Could you check a few things on this model? Use its own coordinates, in mm. A direction names the side the tool comes from. Coordinates: 2 decimals unless noted, no trailing zeros. Order: outer loops, then holes, each group sorted by start corner. A loop starts at its lowest first (then second) coordinate and runs counter-clockwise, first axis right, second up. Notation, with made-up numbers: (-12, 81) - (6, 81) arc R34 cw to (6, 114) - close; hole circle Ø8 at (45.25, 43.25). An arc over 180 degrees is marked (long way). Answer as a JSON object with one key per item and string values. Group by question number.
(1) Imagine slicing it at B-B, the plane x = 0. Write out the boundary of the cut face in (y, z), and give its area (4 significant figures).
(2) Which directions (+Z, -Z, +X, -X, +Y, -Y) give clear straight access to the entire face, cutting with the end or side of a thin tool? Please do faces 5 (the flat face through (0, 1, 3.9)), 6 (the flat face through (8, 1, 5.5)), 7 (the flat face through (-10, 1, -7)).
(3) Imagine slicing it at A-A, the plane z = 0. Write out the boundary of the cut face in (x, y), and give its area (4 significant figures).
(4) Please list where these lines run through material, in increasing order: probe 1 along Z at (x, y) = (-8, -23.5); probe 2 along Z at (x, y) = (9, 34.5); probe 3 along X at (y, z) = (-0.5, 0).
(5) Will these pins go through, and if not, where does the flat tip stop? P1, Ø1.5, axis at x = 0, z = 0, coming from the -Y side; P2, Ø1, axis at x = 2, y = -11, coming from the -Z side.
(6) We'd pull the mould along X, two halves only. Please class faces 1 (the flat face through (2, -57.5, -2)), 2 (the flat face through (-10, 1, 7)), 3 (the flat face through (10, 1, 7)), 4 (the flat face through (5.25, 0.8, 4.19)): pulls with the +X half, pulls with the -X half, needs draft (parallel to the pull), parting line crosses it, or undercut.
from build123d import *

# Parameters (mm, degrees)
SKETCH1_R           = 2.55
BOSS_EXTRUDE1_DEPTH = 57.5


with BuildPart() as part:
    # Sketch1 → Boss-Extrude1 (new, symmetric)
    with BuildSketch(Plane(origin=(0, 0, 0), x_dir=(1, 0, 0), z_dir=(0, 1, 0))):
        Polygon((-6.560660172, 5.5), (-3.9, 2.839339828), (-3.9, -2.839339828), (-6.560660172, -5.5), (-8.5, -5.5), (-8.5, -3.1), (-9.639683838, -3.1), (-9.639683838, -3.65), (-10, -3.65), (-10, -10), (-3.65, -10), (-3.65, -9.639683838), (-3.1, -9.639683838), (-3.1, -8.5), (-5.5, -8.5), (-5.5, -6.560660172), (-2.839339828, -3.9), (2.839339828, -3.9), (5.5, -6.560660172), (5.5, -8.5), (3.1, -8.5), (3.1, -9.639683838), (3.65, -9.639683838), (3.65, -10), (10, -10), (10, -3.65), (9.639683838, -3.65), (9.639683838, -3.1), (8.5, -3.1), (8.5, -5.5), (6.560660172, -5.5), (3.9, -2.839339828), (3.9, 2.839339828), (6.560660172, 5.5), (8.5, 5.5), (8.5, 3.1), (9.639683838, 3.1), (9.639683838, 3.65), (10, 3.65), (10, 10), (3.65, 10), (3.65, 9.639683838), (3.1, 9.639683838), (3.1, 8.5), (5.5, 8.5), (5.5, 6.560660172), (2.839339828, 3.9), (-2.839339828, 3.9), (-5.5, 6.560660172), (-5.5, 8.5), (-3.1, 8.5), (-3.1, 9.639683838), (-3.65, 9.639683838), (-3.65, 10), (-10, 10), (-10, 3.65), (-9.639683838, 3.65), (-9.639683838, 3.1), (-8.5, 3.1), (-8.5, 5.5), align=None)
        with Locations(Location((0, 0, 0), (0, 0, 270))):
            Circle(SKETCH1_R, mode=Mode.SUBTRACT)
    extrude(amount=BOSS_EXTRUDE1_DEPTH, both=True)


solid = part.part
Result set:
{
 "1": {"outline": "(-57.5, -3.9) - (57.5, -3.9) - (57.5, -2.55) - (-57.5, -2.55) - close; (-57.5, 2.55) - (57.5, 2.55) - (57.5, 3.9) - (-57.5, 3.9) - close", "area": "310.5 mm^2"},
 "2": {"face 5": "+Z, +Y, -Y", "face 6": "+Y, -Y", "face 7": "+Z, -Z, -X, +Y, -Y"},
 "3": {"outline": "(-3.9, -57.5) - (-2.55, -57.5) - (-2.55, 57.5) - (-3.9, 57.5) - close; (2.55, -57.5) - (3.9, -57.5) - (3.9, 57.5) - (2.55, 57.5) - close", "area": "310.5 mm^2"},
 "4": {"probe 1": "z = -10 to -5.5, 5.5 to 10", "probe 2": "z = -10 to -3.1, 3.1 to 10", "probe 3": "x = -3.9 to -2.55, 2.55 to 3.9"},
 "5": {"P1": "passes through", "P2": "stops at z = -3.9"},
 "6": {"face 1": "needs draft", "face 2": "pulls with the -X half", "face 3": "pulls with the +X half", "face 4": "undercut"}
}
